The model under review builds one solid part; all positions refer to its coordinate system, in mm. A direction names the side the tool comes from. Give positions to 0.01 mm unless a question says otherwise; leave off trailing zeros. Order: outer loops, then holes, each group sorted by start corner. A loop starts at its lowest first (then second) coordinate and runs counter-clockwise, first axis right, second up. Notation, with made-up numbers: (83.5, -34.75) - (107.5, -34.75) arc R24 ccw to (107.5, 1.25) - close; hole circle Ø2 at (-27.5, 76). An arc over 180 degrees is marked (long way). Write item = value, one per line. Start each with the question number.
1. Mouldability with a two-part tool opening along Y and no side actions: class faces 1 (the flat face through (-22, 88, -4)), 2 (the cylindrical face through (-31.77, -5.37, -1.19)), 3 (the cylindrical face through (-22.12, 78.34, -0.37)) as pulls with the +Y half, pulls with the -Y half, needs draft (parallel to the pull), parting line crosses it, or undercut.
2. We need section A-A, the plane y = 80. Give the boundary of the cut face in (x, z) (3 decimals), and give its area (3 significant figures).
3. We need section D-D, the plane y = 91.5. Give the boundary of the cut face in (x, z) (3 decimals).
4. Wall thickness on probe 1 along Y at (x, z) = (-20.75, -0.75); probe 2 along Z at (x, y) = (-22.2, 95); probe 3 along Z at (x, y) = (-24.75, 0): over which ranges is each line inside the solid? List them lowest first.
5. For P1, Ø4, axis at x = -24.5, y = 53, coming from the -Z side; P2, Ø3, axis at x = -23, y = 83, coming from the -Z side; P3, Ø4, axis at y = 0, z = 0, coming from the +X side (3 decimals); P4, Ø3, axis at y = 80, z = 0, coming from the +X side, all flat-tipped, find the tip position at first contact; note any pin that passes through.
6. Machinability: for faces 4 (the flat face through (-22, 87, 4)), 5 (the flat face through (-22, 100, 0)), 6 (the flat face through (-27.145, 0, 0)), 7 (the cylindrical face through (-22.117, 48.433, 0.221)), 8 (the cylindrical face through (-31.774, -1.341, 3.233)), which of the approach directions +Z, -Z, +X, -X, +Y, -Y give a long, thin tool a straight path to every point of the face, cutting with its end or side? Answer none if there is none.
7. We need section B-B, the plane x = -22. Give the boundary of the cut face in (y, z), and give its area (3 significant figures).
from build123d import *

# Parameters (mm, degrees)
SKETCH1_R           = 7
SKETCH1_R_2         = 3.0845
BOSS_EXTRUDE1_DEPTH = 10
BOSS_EXTRUDE2_START = 7
SKETCH1_3_R         = 7
BOSS_EXTRUDE2_DEPTH = 3
SKETCH1_5_R         = 1.7
BOSS_EXTRUDE3_DEPTH = 4
SKETCH2_R           = 5.5
SKETCH2_R_2         = 3.5
BOSS_EXTRUDE4_DEPTH = 3.305
SKETCH3_R           = 1.7
CUT_EXTRUDE1_DEPTH  = 4


with BuildPart() as part:
    # Sketch1 → Boss-Extrude1 (new body)
    with BuildSketch(Plane.ZY.offset(20.145)):
        Circle(SKETCH1_R)
        Circle(SKETCH1_R_2, mode=Mode.SUBTRACT)
    extrude(amount=BOSS_EXTRUDE1_DEPTH)

    # Sketch1<3> → Boss-Extrude2 (add)
    with BuildSketch(Plane.ZY.offset(20.145).offset(BOSS_EXTRUDE2_START)):
        Circle(SKETCH1_3_R)
    extrude(amount=BOSS_EXTRUDE2_DEPTH)

    # Sketch1<5> → Boss-Extrude3 (add)
    with BuildSketch(Plane.ZY.offset(20.145)):
        with BuildLine():
            Line((-5, 75), (-5, 27.967015644))
            Line((-5, 27.967015644), (-9.925953163, 9.583108165))
            Line((-9.925953163, 9.583108165), (-6.744787083, -1.872924772))
            ThreePointArc((-6.744787083, -1.872924772), (-5.652422268, 4.129179399), (-0.2666949, 6.994917714))
            Line((-0.2666949, 6.994917714), (5, 26.650490668))
            Line((5, 26.650490668), (5, 75))
            Line((5, 75), (4, 75))
            Line((4, 75), (4, 100))
            Line((4, 100), (-4, 100))
            Line((-4, 100), (-4, 75))
            Line((-4, 75), (-5, 75))
        make_face()
        with Locations((0, 80)):
            Circle(SKETCH1_5_R, mode=Mode.SUBTRACT)
        with Locations((0, 95)):
            Circle(SKETCH1_5_R, mode=Mode.SUBTRACT)
    extrude(amount=BOSS_EXTRUDE3_DEPTH)

    # Sketch2 → Boss-Extrude4 (add)
    with BuildSketch(Plane.ZY.offset(30.145)):
        Circle(SKETCH2_R)
        Circle(SKETCH2_R_2, mode=Mode.SUBTRACT)
    extrude(amount=BOSS_EXTRUDE4_DEPTH)

    # Sketch3 → Cut-Extrude1 (cut)
    with BuildSketch(Plane(origin=(-20.145, 0, 0), x_dir=(0, 0, -1), z_dir=(1, 0, 0))):
        with Locations((0, 46.747966087)):
            Circle(SKETCH3_R)
        with Locations((0, 56.747966087)):
            Circle(SKETCH3_R)
    extrude(amount=-CUT_EXTRUDE1_DEPTH, mode=Mode.SUBTRACT)


solid = part.part
Model answer:
q1.face_1 = needs draft
q1.face_2 = parting line crosses it
q1.face_3 = undercut
q2.outline = (-24.145, -4) - (-20.145, -4) - (-20.145, -1.7) - (-24.145, -1.7) - close; (-24.145, 1.7) - (-20.145, 1.7) - (-20.145, 4) - (-24.145, 4) - close
q2.area = 18.4 mm2
q3.outline = (-24.145, -4) - (-20.145, -4) - (-20.145, 4) - (-24.145, 4) - close
q4.probe_1 = -6.96 to -2.99, 2.99 to 45.22, 48.27 to 55.22, 58.27 to 78.47, 81.53 to 93.47, 96.53 to 100
q4.probe_2 = -4 to -1.7, 1.7 to 4
q4.probe_3 = -7 to -3.08, 3.08 to 7
q5.P1 = -5
q5.P2 = -4
q5.P3 = -27.145
q5.P4 = through
q6.face_4 = +Z, +X, -X, +Y
q6.face_5 = +Z, -Z, +X, -X, +Y
q6.face_6 = +X
q6.face_7 = +X, -X
q6.face_8 = -X
q7.outline = (-1.87, -6.74) - (9.58, -9.93) - (27.97, -5) - (75, -5) - (75, -4) - (100, -4) - (100, 4) - (75, 4) - (75, 5) - (26.65, 5) - (6.99, -0.27) arc R7 ccw (long way) to start; hole circle Ø6.17 at (0, 0); hole circle Ø3.4 at (46.75, 0); hole circle Ø3.4 at (56.75, 0); hole circle Ø3.4 at (80, 0); hole circle Ø3.4 at (95, 0)
q7.area = 992 mm2
